Geometry: see drawing. Coordinates: mm, zero at the bounding-box minimum. Coordinates: 2 decimals unless noted, no trailing zeros. Loops run counter-clockwise (first coordinate to the right, second up) from the corner with the lowest first, then second, coordinate; pieces in that order, holes last. Notation, with made-up numbers: (-29.5, 2) -> (21.5, 2) arc R15 ccw to (21.5, 19) -> close; hole circle Ø10 at (45.25, 52.25). An arc over 180 degrees is marked (long way). Put each result on its own line as item: value. Start each with the question number.
1) Pull-direction query (Z, two-part tool) for the marked faces 1 and 2; classes: pulls with the +Z half, pulls with the -Z half, needs draft (parallel to the pull), parting line crosses it, or undercut.
2) Cut plane A-A (y = 3). Return the cut outline in (x, z).
3) Contact query for flat-ended pins moving along their axis: P1, Ø1.5, axis at x = 29.5, y = 3, coming from the +Z side; P2, Ø4, axis at x = 18.5, y = 2.5, coming from the -Z side; P3, Ø2.5, axis at y = 3, z = 43, coming from the +X side. Output: stop coordinate, or through.
4) Material intervals for L1, parallel to Z at x = 23, y = 1.75; L2, parallel to Y at x = 36, z = 20; L3, parallel to X at y = 2.75, z = 73.5, sorted ascending.
5) Cut plane B-B (x = 4). Return the cut outline in (y, z), plus the area to 3 significant figures.
6) Cut plane C-C (z = 32.5). Return the cut outline in (x, y).
7) Cut plane D-D (x = 53). Return the cut outline in (y, z).
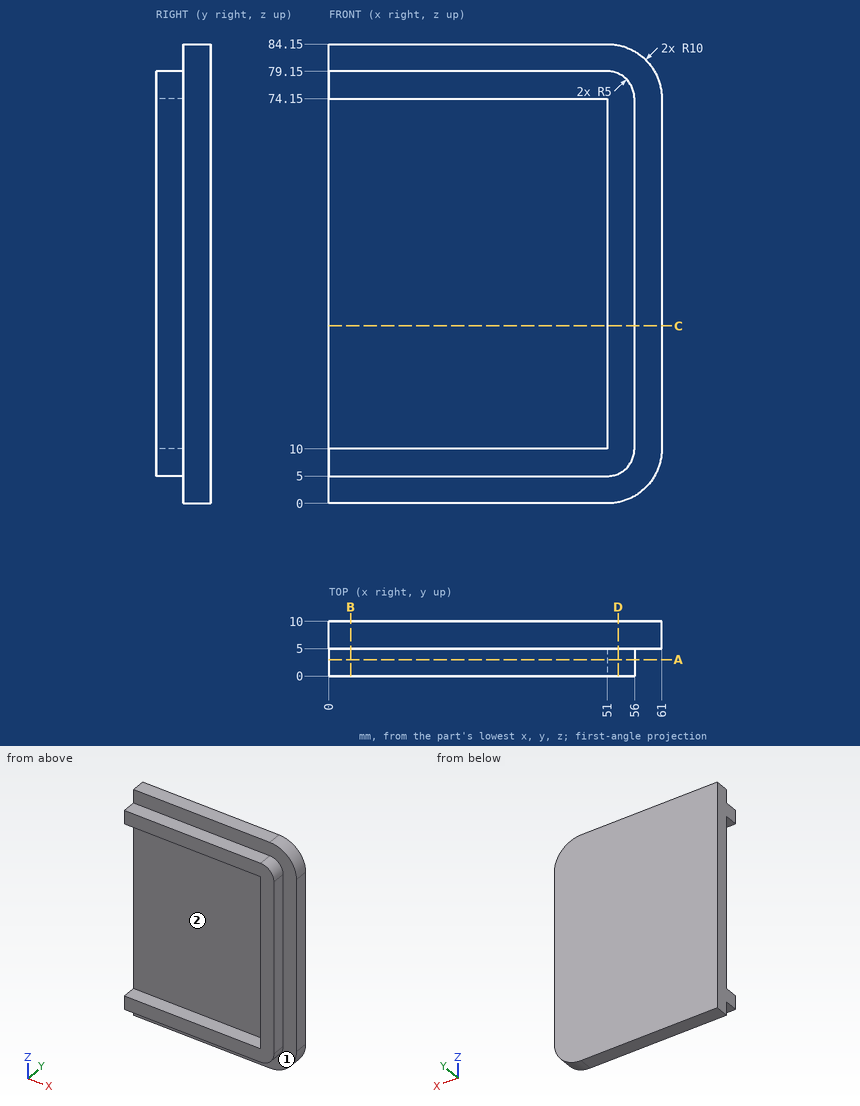
Results found:
1. face 1: needs draft
1. face 2: undercut
2. outline: (0, 5) -> (51, 5) arc R5 ccw to (56, 10) -> (56, 74.15) arc R5 ccw to (51, 79.15) -> (0, 79.15) -> (0, 74.15) -> (51, 74.15) -> (51, 10) -> (0, 10) -> close
3. P1: stops at z = 79.15
3. P2: stops at z = 5
3. P3: stops at x = 56
4. L1: z = 5 to 10, 74.15 to 79.15
4. L2: y = 5 to 10
4. L3: x = 51 to 56
5. outline: (0, 5) -> (5, 5) -> (5, 0) -> (10, 0) -> (10, 84.15) -> (5, 84.15) -> (5, 79.15) -> (0, 79.15) -> (0, 74.15) -> (5, 74.15) -> (5, 10) -> (0, 10) -> close
5. area: 471 mm2
6. outline: (0, 5) -> (51, 5) -> (51, 0) -> (56, 0) -> (56, 5) -> (61, 5) -> (61, 10) -> (0, 10) -> close
7. outline: (0, 5.42) -> (5, 5.42) -> (5, 0.2) -> (10, 0.2) -> (10, 83.95) -> (5, 83.95) -> (5, 78.73) -> (0, 78.73) -> close
